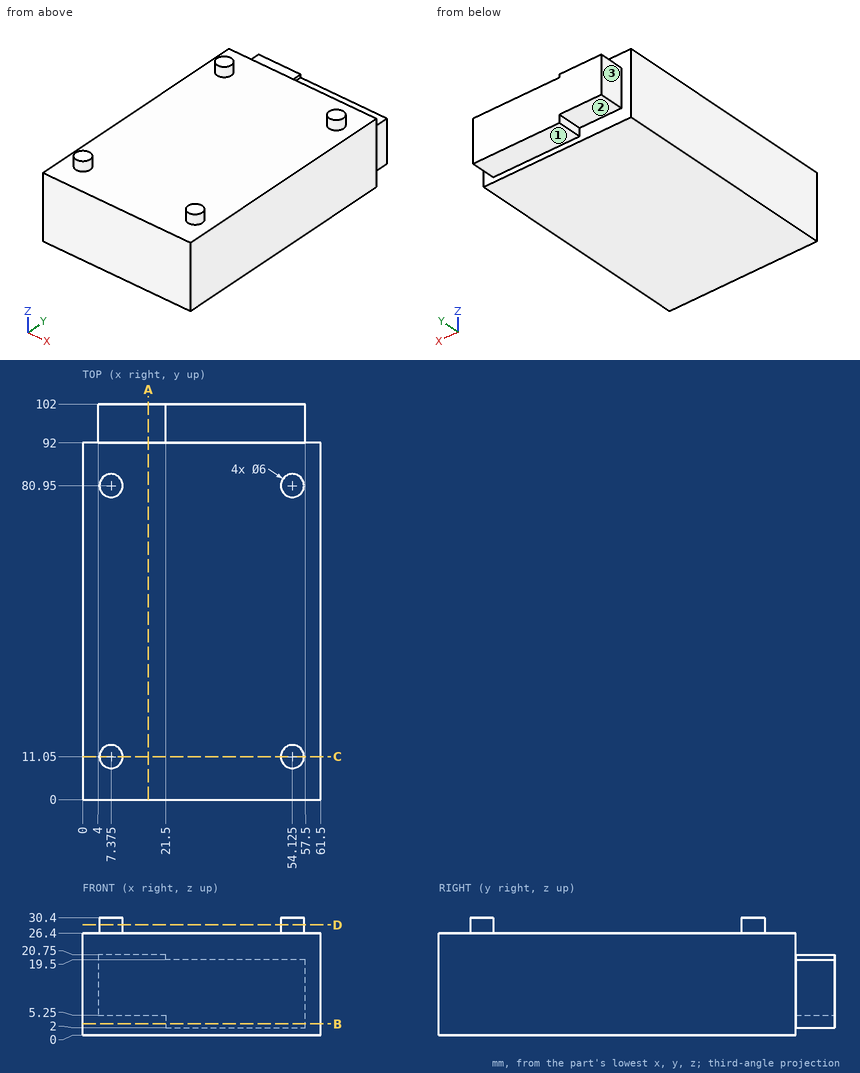
Study the drawing (mm; zero at the part's minimum x, y, z) and answer. A direction names the side the tool comes from. Round coordinates to 2 decimals unless told otherwise and drop trailing zeros. Order: outer loops, then holes, each group sorted by start corner. A loop starts at its lowest first (then second) coordinate and runs counter-clockwise, first axis right, second up. Notation, with made-up numbers: (4, -24) - (39, -24) arc R17 ccw to (39, -4) - close; hole circle Ø4 at (58.25, 35.5). An arc over 180 degrees is marked (long way). Use one line per item in the form item = value. Start each with the question number.
(1) The part is cut by section D-D (z = 28.5). Give the vertices of the cut face in (x, y) (3 decimals), then the cut area to 3 significant figures.
(2) For the marked faces 1, 2 and 3, determine the directions among +Z, -Z, +X, -X, +Y, -Y from which every point of the face is accessible in a straight line to the end or side of a thin tool.
(3) The part is cut by section B-B (z = 3). Give the vertices of the cut face in (x, y).
(4) Flat-ended cylindrical pins translate along their axes: pin 1 Ø18.5 at (x, y) = (30, 53.5) entering from +Z; pin 2 Ø2 at (x, z) = (33, 24) entering from +Y; pin 3 Ø3 at (x, y) = (44, 94.5) entering from -Z. Find the tip coordinate at first contact, or state that the pin passes through.
(5) The part is cut by section C-C (y = 11.05). Give the vertices of the cut face in (x, z) (3 decimals), then the cut area to 3 significant figures.
(6) The part is cut by section A-A (x = 17). Give the vertices of the cut face in (y, z).
(7) Find the intervals of material crossed by line 1 along Z through (x, y) = (6.5, 52.5); line 2 along Y through (x, z) = (58.5, 6.5), in increasing order. Write a range as from..to.
Checked values:
q1.outline = circle Ø6 at (7.375, 11.05); circle Ø6 at (7.375, 80.95); circle Ø6 at (54.125, 11.05); circle Ø6 at (54.125, 80.95)
q1.area = 113 mm^2
q2.face_1 = -Z, +X, -X, +Y
q2.face_2 = -Z, -X, +Y
q2.face_3 = +Z, -Z, -X, +Y
q3.outline = (0, 0) - (61.5, 0) - (61.5, 92) - (57.5, 92) - (57.5, 102) - (21.5, 102) - (21.5, 92) - (0, 92) - close
q4.pin_1 = 26.4
q4.pin_2 = 92
q4.pin_3 = 2
q5.outline = (0, 0) - (61.5, 0) - (61.5, 26.4) - (57.125, 26.4) - (57.125, 30.4) - (51.125, 30.4) - (51.125, 26.4) - (10.375, 26.4) - (10.375, 30.4) - (4.375, 30.4) - (4.375, 26.4) - (0, 26.4) - close
q5.area = 1,670 mm^2
q6.outline = (0, 0) - (92, 0) - (92, 5.25) - (102, 5.25) - (102, 20.75) - (92, 20.75) - (92, 26.4) - (0, 26.4) - close
q7.line_1 = 0..26.4
q7.line_2 = 0..92
